Model file for the job. Use its own axes, mm. Face numbers are marked on the shaded views. A direction names the side the tool comes from. Round coordinates to 2 decimals unless told otherwise and drop trailing zeros. Loops run counter-clockwise (first coordinate to the right, second up) from the corner with the lowest first, then second, coordinate; pieces in that order, holes last. Notation, with made-up numbers: M -2,84.25 L 12,84.25 A29 ccw 12,105.25 Z; hole C 57.25,-19.75 d5. An arc over 180 degrees is marked long. Use a Markdown table: item, result. Add a question column.
Item 1: Pin check, flat tips, straight feed: P1, Ø12, axis at y = 2.5, z = -21.5, coming from the +X side; P2, Ø3.5, axis at y = 5, z = -21.5, coming from the -X side; P3, Ø5, axis at x = 12.5, z = -47.5, coming from the +Y side. Stop position of each tip, or through.
Item 2: Tool access for the marked faces 4, 5 and 6: list every direction of +Z, -Z, +X, -X, +Y, -Y with a clear straight run to the whole face (end or side of a thin tool).
Item 3: Saw through at A-A on y = 12.25. Write the cut outline in (x, z), then the cut area to 3 significant figures.
Item 4: Wall check: L1, parallel to X at y = 11.85, z = -27; L2, parallel to Z at x = 27, y = 13.1; L3, parallel to Z at x = 19, y = 1.5. Give the ranges that are in metal, low to high. Write a range as from..to.
Item 5: Two-plate mould, pull along X, no slides. Class the marked faces 1, 2 and 3: +X half, -X half, draft (parallel to the pull), parting line (faces both ways), or undercut.
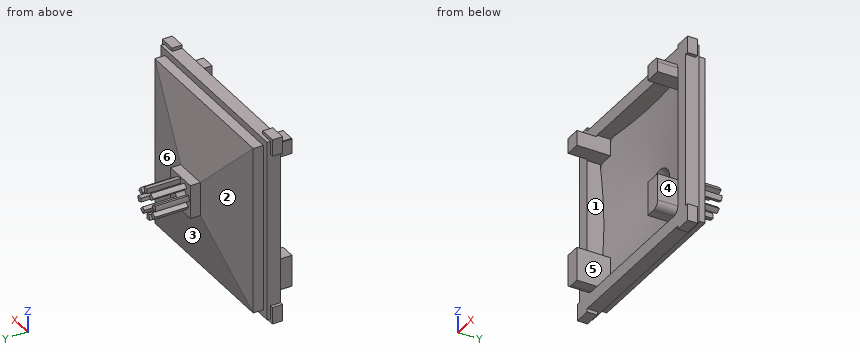
```python
from build123d import *
from build123d.topology import SkipClean

# Parameters (mm, degrees)
SKETCH_1_W          = 54
SKETCH_1_H          = 54
EXTRUDE_1_DEPTH     = 4
SKETCH_2_W          = 50
SKETCH_2_H          = 50
EXTRUDE_2_DEPTH     = 8
CHAMFER_1_SIZE      = 5
CHAMFER_1_SIZE_2    = 25
SKETCH_3_W          = 56
SKETCH_3_H          = 56
EXTRUDE_3_DEPTH     = 3
SKETCH_4_W          = 46
SKETCH_4_H          = 1
SKETCH_4_W_2        = 1
SKETCH_4_H_2        = 46
CUT_EXTRUDE_1_DEPTH = 3
EXTRUDE_START       = 10
SKETCH_5_W          = 10
SKETCH_5_H          = 10
EXTRUDE_4_DEPTH     = 4
EXTRUDE_5_DEPTH     = 10
SKETCH_10_W         = 46
SKETCH_10_H         = 46
CUT_EXTRUDE_2_DEPTH = 4
SKETCH_12_R         = 3
CUT_EXTRUDE_3_DEPTH = 15
CHAMFER_2_SIZE      = 5
CHAMFER_2_SIZE2     = 7.140740034
CHAMFER_3_SIZE      = 5
CHAMFER_3_SIZE_2    = 20.3603283
SKETCH_13_W         = 5
SKETCH_13_H         = 5
EXTRUDE_6_DEPTH     = 10
SKETCH_14_W         = 5
SKETCH_14_H         = 10
EXTRUDE_7_DEPTH     = 10
FILLET_1_R          = 2
CUT_EXTRUDE_4_DEPTH = 6
SKETCH_16_W         = 12.181950641
SKETCH_16_H         = 4.017842963
CUT_EXTRUDE_5_DEPTH = 82.012344772


with BuildPart() as part:
    # Эскиз1 → Бобышка-Вытянуть1 (new body)
    with BuildSketch(Plane(origin=(0, 0, 0), x_dir=(1, 0, 0), z_dir=(0, 1, 0))):
        with Locations((27, 27)):
            Rectangle(SKETCH_1_W, SKETCH_1_H)
    extrude(amount=EXTRUDE_1_DEPTH)

    # Эскиз2 → Бобышка-Вытянуть2 (add)
    with BuildSketch(Plane(origin=(0, 4, 0), x_dir=(1, 0, 0), z_dir=(0, 1, 0))):
        with Locations((27, 27)):
            Rectangle(SKETCH_2_W, SKETCH_2_H)
    extrude(amount=EXTRUDE_2_DEPTH)

    # Фаска1
    # the kernel refuses this chamfer: 25, 5 mm, written as the material it takes off along each edge
    with BuildSketch(Plane(origin=(2, 12, -116.953302157), x_dir=(-0.18544098588999025, -0.9826554028509427, 0), z_dir=(0, 0, 1)), Plane(origin=(-62.953302157, 12, -2), x_dir=(0, -0.9826554028509427, 0.18544098588999025), z_dir=(1, 0, 0)), Plane(origin=(52, 12, 62.953302157), x_dir=(0.18544098588999086, -0.9826554028509427, 0), z_dir=(0, 0, -1)), Plane(origin=(116.953302157, 12, -52), x_dir=(0, -0.9826554028509427, -0.18544098588999086), z_dir=(-1, 0, 0))) as chamfer_1_piece_1:
        Polygon((CHAMFER_1_SIZE * 0.982655402851, CHAMFER_1_SIZE * 0.18544098589), (-CHAMFER_1_SIZE_2 * 0.18544098589, CHAMFER_1_SIZE_2 * 0.982655402851), (0, 0), align=None)
    extrude(amount=179.906604315, mode=Mode.SUBTRACT)

    # Эскиз3 → Бобышка-Вытянуть3 (add)
    with BuildSketch(Plane(origin=(0, 0, 0), x_dir=(1, 0, 0), z_dir=(0, 1, 0))):
        with Locations((27, 27)):
            Rectangle(SKETCH_3_W, SKETCH_3_H)
    extrude(amount=EXTRUDE_3_DEPTH)

    # Эскиз4 → Вырез-Вытянуть1 (cut)
    with BuildSketch(Plane(origin=(0, 3, 0), x_dir=(1, 0, 0), z_dir=(0, 1, 0))):
        with Locations((27, 54.5)):
            Rectangle(SKETCH_4_W, SKETCH_4_H)
        with Locations((-0.5, 27)):
            Rectangle(SKETCH_4_W_2, SKETCH_4_H_2)
        with Locations((54.5, 27)):
            Rectangle(SKETCH_4_W_2, SKETCH_4_H_2)
        with Locations((27, -0.5)):
            Rectangle(SKETCH_4_W, SKETCH_4_H)
    extrude(amount=-CUT_EXTRUDE_1_DEPTH, mode=Mode.SUBTRACT)

    # Эскиз5 → Бобышка-Вытянуть4 (add)
    with BuildSketch(Plane(origin=(0, 0, 0), x_dir=(1, 0, 0), z_dir=(0, 1, 0)).offset(EXTRUDE_START)):
        with Locations((27, 27)):
            Rectangle(SKETCH_5_W, SKETCH_5_H)
    extrude(amount=EXTRUDE_4_DEPTH)

    # Эскиз6 → Бобышка-Вытянуть5 (add)
    with BuildSketch(Plane(origin=(0, 14, 0), x_dir=(1, 0, 0), z_dir=(0, 1, 0))):
        with BuildLine():
            Line((27, 30), (27, 31.5))
            ThreePointArc((27, 31.5), (26.2185832, 31.431634889), (25.460909355, 31.228616794))
            Line((25.460909355, 31.228616794), (25.97393957, 29.819077862))
            ThreePointArc((25.97393957, 29.819077862), (26.479055467, 29.954423259), (27, 30))
        make_face()
        with BuildLine():
            Line((29.121320344, 29.121320344), (30.181980515, 30.181980515))
            ThreePointArc((30.181980515, 30.181980515), (29.581093964, 30.686184199), (28.901782178, 31.078385042))
            Line((28.901782178, 31.078385042), (28.267854785, 29.718923361))
            ThreePointArc((28.267854785, 29.718923361), (28.720729309, 29.457456133), (29.121320344, 29.121320344))
        make_face()
        with BuildLine():
            Line((30, 27), (31.5, 27))
            ThreePointArc((31.5, 27), (31.431634889, 27.7814168), (31.228616794, 28.539090645))
            Line((31.228616794, 28.539090645), (29.819077862, 28.02606043))
            ThreePointArc((29.819077862, 28.02606043), (29.954423259, 27.520944533), (30, 27))
        make_face()
        with BuildLine():
            Line((29.121320344, 24.878679656), (30.181980515, 23.818019485))
            ThreePointArc((30.181980515, 23.818019485), (30.686184199, 24.418906036), (31.078385042, 25.098217822))
            Line((31.078385042, 25.098217822), (29.718923361, 25.732145215))
            ThreePointArc((29.718923361, 25.732145215), (29.457456133, 25.279270691), (29.121320344, 24.878679656))
        make_face()
        with BuildLine():
            Line((27, 24), (27, 22.5))
            ThreePointArc((27, 22.5), (27.7814168, 22.568365111), (28.539090645, 22.771383206))
            Line((28.539090645, 22.771383206), (28.02606043, 24.180922138))
            ThreePointArc((28.02606043, 24.180922138), (27.520944533, 24.045576741), (27, 24))
        make_face()
        with BuildLine():
            Line((24.878679656, 24.878679656), (23.818019485, 23.818019485))
            ThreePointArc((23.818019485, 23.818019485), (24.418906036, 23.313815801), (25.098217822, 22.921614958))
            Line((25.098217822, 22.921614958), (25.732145215, 24.281076639))
            ThreePointArc((25.732145215, 24.281076639), (25.279270691, 24.542543867), (24.878679656, 24.878679656))
        make_face()
        with BuildLine():
            Line((24, 27), (22.5, 27))
            ThreePointArc((22.5, 27), (22.568365111, 26.2185832), (22.771383206, 25.460909355))
            Line((22.771383206, 25.460909355), (24.180922138, 25.97393957))
            ThreePointArc((24.180922138, 25.97393957), (24.045576741, 26.479055467), (24, 27))
        make_face()
        with BuildLine():
            Line((24.878679656, 29.121320344), (23.818019485, 30.181980515))
            ThreePointArc((23.818019485, 30.181980515), (23.313815801, 29.581093964), (22.921614958, 28.901782178))
            Line((22.921614958, 28.901782178), (24.281076639, 28.267854785))
            ThreePointArc((24.281076639, 28.267854785), (24.542543867, 28.720729309), (24.878679656, 29.121320344))
        make_face()
    extrude(amount=EXTRUDE_5_DEPTH)

    # Эскиз9 → Повернуть1 (revolve)
    with BuildSketch(Plane(origin=(27, 0, 0), x_dir=(0, 0, -1), z_dir=(1, 0, 0))):
        with BuildLine():
            Line((27, 24), (33, 24))
            Line((33, 24), (28.599558116, 25.80595603))
            ThreePointArc((28.599558116, 25.80595603), (27.95267314, 26.60779708), (27, 27))
            Line((27, 27), (27, 24))
        make_face()
    revolve(axis=Axis((27, 24, -27), (0, 1, 0)))

    # Эскиз10 → Вырез-Вытянуть2 (cut)
    with BuildSketch(Plane(origin=(0, 0, 0), x_dir=(1, 0, 0), z_dir=(0, 1, 0))):
        with Locations((27, 27)):
            Rectangle(SKETCH_10_W, SKETCH_10_H)
    extrude(amount=CUT_EXTRUDE_2_DEPTH, mode=Mode.SUBTRACT)

    # Эскиз12 → Вырез-Вытянуть3 (cut)
    with SkipClean():  # the faces are left unmerged after this step: merging them gives an invalid solid
        with BuildSketch(Plane(origin=(0, 0, 0), x_dir=(1, 0, 0), z_dir=(0, 1, 0))):
            with Locations(Location((27, 27, 0), (0, 0, 270))):
                Circle(SKETCH_12_R)
        extrude(amount=CUT_EXTRUDE_3_DEPTH, mode=Mode.SUBTRACT)
    add(part.part.scale(1), mode=Mode.REPLACE)  # the faces are merged on a copy

    # Фаска2
    chamfer_2_edges = [part.edges().sort_by_distance(p)[0] for p in [
        (27, 4, -30),
    ]]
    chamfer_2_side = [part.faces().sort_by_distance(p)[0] for p in [
        (27, 4, -49.349461761),
    ]]
    chamfer(chamfer_2_edges, length=CHAMFER_2_SIZE, length2=CHAMFER_2_SIZE2, reference=chamfer_2_side[0])

    # Фаска3
    # the kernel refuses this chamfer: 20.3603283, 5 mm, written as the material it takes off along each edge
    with BuildSketch(Plane(origin=(27, 4, -27), x_dir=(0, 0, 1), z_dir=(1, 0, 0))) as chamfer_3_piece_1_section:
        Polygon((8 - CHAMFER_3_SIZE * 0.573576436351, -CHAMFER_3_SIZE * 0.819152044289), (8 + CHAMFER_3_SIZE_2, 0), (8, 0), align=None)
    chamfer_3_piece_1 = revolve(axis=Axis((27, 4, -27), (0, -1, 0)), mode=Mode.PRIVATE)
    chamfer_3_piece_1 = split(chamfer_3_piece_1, bisect_by=Plane(origin=(27, 5.887283675, -50), z_dir=(0, 0, 1)), keep=Keep.TOP, mode=Mode.PRIVATE)
    chamfer_3_piece_1 = split(chamfer_3_piece_1, bisect_by=Plane(origin=(4, 5.887283675, -43.717905574), z_dir=(1, 0, 0)), keep=Keep.TOP, mode=Mode.PRIVATE)
    chamfer_3_piece_1 = split(chamfer_3_piece_1, bisect_by=Plane(origin=(50, 5.887283675, -43.717905574), z_dir=(-1, 0, 0)), keep=Keep.TOP, mode=Mode.PRIVATE)
    chamfer_3_piece_1 = split(chamfer_3_piece_1, bisect_by=Plane(origin=(27, 5.887283675, -4), z_dir=(0, 0, -1)), keep=Keep.TOP, mode=Mode.PRIVATE)
    add(chamfer_3_piece_1, mode=Mode.SUBTRACT)

    # Эскиз13 → Бобышка-Вытянуть6 (add)
    with SkipClean():  # the faces are left unmerged after this step: merging them gives an invalid solid
        with BuildSketch(Plane.XZ.offset(-4)):
            with Locations((6.5, -6.5)):
                Rectangle(SKETCH_13_W, SKETCH_13_H)
            with Locations((47.5, -6.5)):
                Rectangle(SKETCH_13_W, SKETCH_13_H)
        extrude(amount=EXTRUDE_6_DEPTH)

    # Эскиз14 → Бобышка-Вытянуть7 (add)
    with SkipClean():  # the faces are left unmerged after this step: merging them gives an invalid solid
        with BuildSketch(Plane.XZ.offset(-4)):
            with Locations((47.5, -45)):
                Rectangle(SKETCH_14_W, SKETCH_14_H)
            with Locations((6.5, -45)):
                Rectangle(SKETCH_14_W, SKETCH_14_H)
        extrude(amount=EXTRUDE_7_DEPTH)

    # Скругление1
    fillet_1_edges = [part.edges().sort_by_distance(p)[0] for p in [
        (4, -3, -4),
        (50, -3, -4),
        (50, -3, -50),
        (4, -3, -50),
    ]]
    fillet(fillet_1_edges, radius=FILLET_1_R)

    # Эскиз15 → Вырез-Вытянуть4 (cut)
    with BuildSketch(Plane.XZ.offset(6)):
        Polygon((51, -4.5), (4.5, -4.5), (4.5, -51), (2.5, -51), (2.5, -2.5), (51, -2.5), align=None)
    extrude(amount=-CUT_EXTRUDE_4_DEPTH, mode=Mode.SUBTRACT)

    # Эскиз16 → Вырез-Вытянуть5 (cut, through all)
    with BuildSketch(Plane.ZY.offset(-2)):
        with Locations((-26.909024679, 26.008921482)):
            Rectangle(SKETCH_16_W, SKETCH_16_H)
    extrude(amount=-CUT_EXTRUDE_5_DEPTH, mode=Mode.SUBTRACT)


solid = part.part
```
Entries:
| question | item | result |
|---|---|---|
| 1 | P1 | x = 54 |
| 1 | P2 | x = 0 |
| 1 | P3 | y = 8.4 |
| 2 | face 4 | +Z, -Z, +X, -Y |
| 2 | face 5 | -Y |
| 2 | face 6 | +Z, -Z, +X, +Y |
| 3 | outline | M 22,-32 L 32,-32 L 32,-22 L 22,-22 Z; hole C 27,-27 d6 |
| 3 | area | 71.7 mm2 |
| 4 | L1 | 22..24, 30..32 |
| 4 | L2 | -32..-30, -24..-22 |
| 4 | L3 | -54..-50, -4..0 |
| 5 | face 1 | undercut |
| 5 | face 2 | -X half |
| 5 | face 3 | draft |
